Study the drawing (mm; zero at the part's minimum x, y, z) and answer. Coordinates: 2 decimals unless noted, no trailing zeros. Write each loop counter-clockwise with the first axis right and the second up, starting at its lowest first coordinate (ties: lowest second). Pieces come first, ordered by that corner, then holes. Notation, with made-up numbers: M 76.5,30.25 L 127.5,30.25 A18 ccw 127.5,52.25 Z; hole C 47,-7.5 d2. An arc over 180 degrees is marked long. Answer as a JSON object with one key per item and string values. Group by question number.
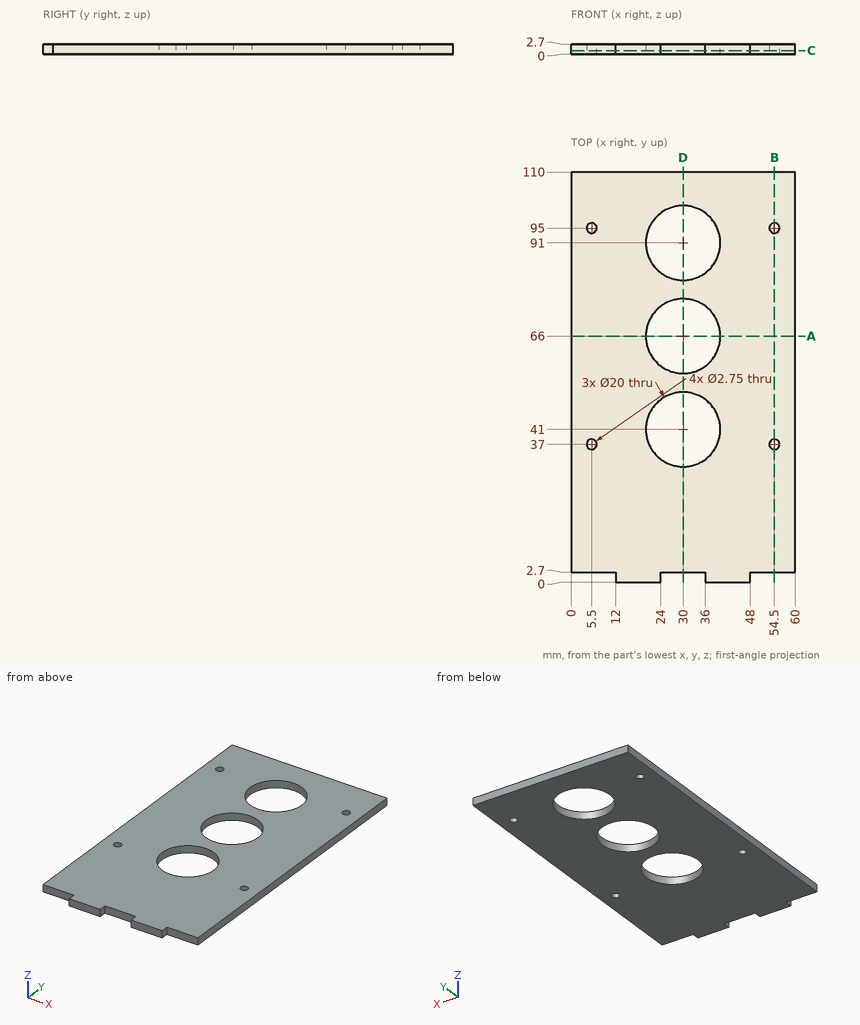
Item 1: A cutting plane is placed at C-C, the plane z = 0.9. Write down the section's boundary in (x, y) (3 decimals), and give its area (3 significant figures).
Item 2: Flat-ended cylindrical pins translate along their axes: pin 1 Ø2 at (x, y) = (54.5, 37) entering from +Z; pin 2 Ø0.8 at (x, z) = (30, 1) entering from -Y; pin 3 Ø1.4 at (y, z) = (1.5, 1.5) entering from +X. Find the tip coordinate at first contact, or state that the pin passes through.
Item 3: A cutting plane is placed at B-B, the plane x = 54.5. Write down the section's boundary in (y, z) (3 decimals).
Item 4: A cutting plane is placed at A-A, the plane y = 66. Write down the section's boundary in (x, z), and give its area (3 significant figures).
Item 5: Consider L1, parallel to Y at x = 30, z = 0.9; L2, parallel to Y at x = 54.5, z = 2.15 (3 decimals); L3, parallel to Y at x = 31, z = 1.05. Determine where each line is inside the solid, lowest interval first. Write a range as from..to.
Item 6: A cutting plane is placed at D-D, the plane x = 30. Write down the section's boundary in (y, z).
Answer:
{
 "1": {"outline": "M 0,2.7 L 12,2.7 L 12,0 L 24,0 L 24,2.7 L 36,2.7 L 36,0 L 48,0 L 48,2.7 L 60,2.7 L 60,110 L 0,110 Z; hole C 5.5,37 d2.75; hole C 5.5,95 d2.75; hole C 30,41 d20; hole C 30,66 d20; hole C 30,91 d20; hole C 54.5,37 d2.75; hole C 54.5,95 d2.75", "area": "5,540 mm2"},
 "2": {"pin 1": "through", "pin 2": "y = 2.7", "pin 3": "x = 48"},
 "3": {"outline": "M 2.7,0 L 35.625,0 L 35.625,2.7 L 2.7,2.7 Z; M 38.375,0 L 93.625,0 L 93.625,2.7 L 38.375,2.7 Z; M 96.375,0 L 110,0 L 110,2.7 L 96.375,2.7 Z"},
 "4": {"outline": "M 0,0 L 20,0 L 20,2.7 L 0,2.7 Z; M 40,0 L 60,0 L 60,2.7 L 40,2.7 Z", "area": "108 mm2"},
 "5": {"L1": "2.7..31, 51..56, 76..81, 101..110", "L2": "2.7..35.625, 38.375..93.625, 96.375..110", "L3": "2.7..31.05, 50.95..56.05, 75.95..81.05, 100.95..110"},
 "6": {"outline": "M 2.7,0 L 31,0 L 31,2.7 L 2.7,2.7 Z; M 51,0 L 56,0 L 56,2.7 L 51,2.7 Z; M 76,0 L 81,0 L 81,2.7 L 76,2.7 Z; M 101,0 L 110,0 L 110,2.7 L 101,2.7 Z"}
}
